from build123d import *

# Parameters (mm, degrees)
BOSS_EXTRUDE1_DEPTH = 18.5
BOSS_EXTRUDE2_DEPTH = 3
BOSS_EXTRUDE3_START = 7
BOSS_EXTRUDE3_DEPTH = 3.5
SKETCH4_W           = 6.5
SKETCH4_H           = 2.25
BOSS_EXTRUDE4_DEPTH = 20
FILLET1_R           = 2.25
BOSS_EXTRUDE5_DEPTH = 7
BOSS_EXTRUDE6_DEPTH = 3
SKETCH7_R           = 2.5
CUT_EXTRUDE1_DEPTH  = 75.541934507
SKETCH8_R           = 2.2
CUT_EXTRUDE2_DEPTH  = 74.11976477
CUT_EXTRUDE3_REACH  = 75.12
SKETCH9_R           = 2.2
BOSS_EXTRUDE7_REACH = 77.196
SKETCH10_R          = 3.5
SKETCH10_R_2        = 2.5
BOSS_EXTRUDE8_REACH = 74.419
SKETCH11_R          = 3.5
SKETCH11_R_2        = 2.5
CUT_EXTRUDE4_REACH  = 66.742
SKETCH12_W          = 7
SKETCH12_H          = 5
CHAMFER1_SIZE       = 1.5


with BuildPart() as part:
    # Sketch1 → Boss-Extrude1 (new body)
    with BuildSketch(Plane(origin=(0, 0, 0), x_dir=(1, 0, 0), z_dir=(0, 1, 0))):
        Polygon((40.5, 0), (0, 0), (0, -58), (3, -58), (3, -3), (40.5, -3), align=None)
    extrude(amount=BOSS_EXTRUDE1_DEPTH)

    # Sketch2 → Boss-Extrude2 (add)
    with BuildSketch(Plane.XZ):
        with BuildLine():
            Line((40.5, 3), (23.5, 19.5))
            Line((23.5, 19.5), (23.5, 37))
            ThreePointArc((23.5, 37), (20.571067812, 44.071067812), (13.5, 47))
            Line((13.5, 47), (3, 47))
            Line((3, 47), (3, 3))
            Line((3, 3), (40.5, 3))
        make_face()
    extrude(amount=-BOSS_EXTRUDE2_DEPTH)

    # Sketch3 → Boss-Extrude3 (add)
    with BuildSketch(Plane(origin=(0, 3, 0), x_dir=(1, 0, 0), z_dir=(0, 1, 0)).offset(BOSS_EXTRUDE3_START)):
        with BuildLine():
            Line((3, -47), (13.5, -47))
            ThreePointArc((13.5, -47), (23.5, -37), (13.5, -27))
            Line((13.5, -27), (3, -27))
            Line((3, -27), (3, -47))
        make_face()
    extrude(amount=BOSS_EXTRUDE3_DEPTH)

    # Sketch4 → Boss-Extrude4 (add)
    with BuildSketch(Plane.XY.offset(47)):
        with Locations((6.25, 14.625)):
            Rectangle(SKETCH4_W, SKETCH4_H)
    extrude(amount=-BOSS_EXTRUDE4_DEPTH)

    # Fillet1
    fillet1_edges = [part.edges().sort_by_distance(p)[0] for p in [
        (9.5, 15.75, 37),
    ]]
    fillet(fillet1_edges, radius=FILLET1_R - 0.0001)  # a hair under: the kernel refuses the full size

    # Sketch5 → Boss-Extrude5 (add)
    with BuildSketch(Plane.XZ):
        Polygon((0, 31.5), (0, 11.5), (9, 11.5), (9, 13.5), (3, 13.5), (3, 31.5), align=None)
    extrude(amount=BOSS_EXTRUDE5_DEPTH)

    # Sketch6 → Boss-Extrude6 (add)
    with BuildSketch(Plane.XZ.offset(7)):
        with BuildLine():
            Line((0, 11.5), (0, 31.5))
            Line((0, 31.5), (13.5, 31.5))
            ThreePointArc((13.5, 31.5), (23.5, 21.5), (13.5, 11.5))
            Line((13.5, 11.5), (0, 11.5))
        make_face()
    extrude(amount=BOSS_EXTRUDE6_DEPTH)

    # Sketch7 → Cut-Extrude1 (cut, through all)
    with BuildSketch(Plane(origin=(0, 13.5, 0), x_dir=(1, 0, 0), z_dir=(0, 1, 0))):
        with Locations(Location((15.5, -21.5, 0), (0, 0, 270))):
            Circle(SKETCH7_R)
        with Locations(Location((15.5, -37, 0), (0, 0, 270))):
            Circle(SKETCH7_R)
    extrude(amount=-CUT_EXTRUDE1_DEPTH, mode=Mode.SUBTRACT)

    # Sketch8 → Cut-Extrude2 (cut, through all)
    with BuildSketch(Plane.ZY):
        with Locations((11, 8.5)):
            Circle(SKETCH8_R)
        with Locations((51.5, 8.5)):
            Circle(SKETCH8_R)
    extrude(amount=-CUT_EXTRUDE2_DEPTH, mode=Mode.SUBTRACT)

    # Sketch9 → Cut-Extrude3 (cut, up to next)
    with BuildSketch(Plane(origin=(0, 0, 0), x_dir=(-1, 0, 0), z_dir=(0, 0, -1)), mode=Mode.PRIVATE) as cut_extrude3_sk1:
        with Locations((-34.5, 8.5)):
            Circle(SKETCH9_R)
    cut_extrude3_tool1 = extrude(cut_extrude3_sk1.sketch, amount=-CUT_EXTRUDE3_REACH, mode=Mode.PRIVATE) & part.part
    # Sketch9 → Cut-Extrude3 (cut, up to next)
    with BuildSketch(Plane(origin=(0, 0, 0), x_dir=(-1, 0, 0), z_dir=(0, 0, -1)), mode=Mode.PRIVATE) as cut_extrude3_sk2:
        with Locations((-11, 8.5)):
            Circle(SKETCH9_R)
    cut_extrude3_tool2 = extrude(cut_extrude3_sk2.sketch, amount=-CUT_EXTRUDE3_REACH, mode=Mode.PRIVATE) & part.part
    add(cut_extrude3_tool1.solids().sort_by_distance((34.5, 8.5, 0))[0], mode=Mode.SUBTRACT)
    add(cut_extrude3_tool2.solids().sort_by_distance((11, 8.5, 0))[0], mode=Mode.SUBTRACT)

    # Sketch10 → Boss-Extrude7 (add, up to next)
    with BuildSketch(Plane(origin=(0, -7, 0), x_dir=(1, 0, 0), z_dir=(0, 1, 0)), mode=Mode.PRIVATE) as boss_extrude7_sk1:
        with Locations(Location((15.5, -21.5, 0), (0, 0, 270))):
            Circle(SKETCH10_R)
        with Locations(Location((15.5, -21.5, 0), (0, 0, 270))):
            Circle(SKETCH10_R_2, mode=Mode.SUBTRACT)
    boss_extrude7_tool1 = extrude(boss_extrude7_sk1.sketch, amount=BOSS_EXTRUDE7_REACH, mode=Mode.PRIVATE) - part.part
    add(boss_extrude7_tool1.solids().sort_by_distance((15.5, -7, 18.098995))[0])

    # Sketch11 → Boss-Extrude8 (add, up to next)
    with BuildSketch(Plane(origin=(0, 3, 0), x_dir=(1, 0, 0), z_dir=(0, 1, 0)), mode=Mode.PRIVATE) as boss_extrude8_sk1:
        with Locations(Location((15.5, -37, 0), (0, 0, 90))):
            Circle(SKETCH11_R)
        with Locations(Location((15.5, -37, 0), (0, 0, 270))):
            Circle(SKETCH11_R_2, mode=Mode.SUBTRACT)
    boss_extrude8_tool1 = extrude(boss_extrude8_sk1.sketch, amount=BOSS_EXTRUDE8_REACH, mode=Mode.PRIVATE) - part.part
    add(boss_extrude8_tool1.solids().sort_by_distance((15.5, 3, 40.401005))[0])

    # Cut-Extrude4: up to this face of the body (flat: up to its plane)
    cut_extrude4_end = Plane(part.part.faces().sort_by_distance((21.694792225, 10.874217494, 3))[0])
    # Sketch12 → Cut-Extrude4 (cut, up to the picked face)
    with BuildSketch(Plane.XY.offset(47), mode=Mode.PRIVATE) as cut_extrude4_sk1:
        with Locations((15.5, -3.5)):
            Rectangle(SKETCH12_W, SKETCH12_H)
    cut_extrude4_tool1 = split(extrude(cut_extrude4_sk1.sketch, amount=-CUT_EXTRUDE4_REACH, mode=Mode.PRIVATE), bisect_by=cut_extrude4_end, keep=Keep.BOTH, mode=Mode.PRIVATE)
    # Sketch12 → Cut-Extrude4 (cut, up to the picked face)
    with BuildSketch(Plane.XY.offset(47), mode=Mode.PRIVATE) as cut_extrude4_sk2:
        with Locations((15.5, 6.5)):
            Rectangle(SKETCH12_W, SKETCH12_H)
    cut_extrude4_tool2 = split(extrude(cut_extrude4_sk2.sketch, amount=-CUT_EXTRUDE4_REACH, mode=Mode.PRIVATE), bisect_by=cut_extrude4_end, keep=Keep.BOTH, mode=Mode.PRIVATE)
    add(cut_extrude4_tool1.solids().sort_by(Axis((15.5, -3.5, 47), (0, 0, -1)))[0], mode=Mode.SUBTRACT)
    add(cut_extrude4_tool2.solids().sort_by(Axis((15.5, 6.5, 47), (0, 0, -1)))[0], mode=Mode.SUBTRACT)

    # Chamfer1
    chamfer1_edges = [part.edges().sort_by_distance(p)[0] for p in [
        (9, -3.5, 13.5),
    ]]
    chamfer(chamfer1_edges, length=CHAMFER1_SIZE)


solid = part.part
Work out the finished part from the listing and answer in its coordinate system (mm). A direction names the side the tool comes from. Coordinates: 2 decimals unless noted, no trailing zeros. Loops run counter-clockwise (first coordinate to the right, second up) from the corner with the lowest first, then second, coordinate; pieces in that order, holes last. Notation, with made-up numbers: M 30.5,43 L 64.5,43 A18 ccw 64.5,57 Z; hole C 52.25,-37.75 d5. An arc over 180 degrees is marked long. Answer in a Markdown table with one row per item. Add a question column.
1. The mould has two halves that part along Y. Classify faces 1 (the cylindrical face through (15.346, 3.493, 40.497)), 2 (the cylindrical face through (8.86, 15.07, 36.86)), 3 (the flat face through (21, 11, 3)): pulls with the +Y half, pulls with the -Y half, needs draft (parallel to the pull), parting line crosses it, or undercut.
2. Flat-ended cylindrical pins translate along their axes: P1, Ø1.5, axis at x = 9, y = 1.5, coming from the +Z side; P2, Ø3, axis at x = 21.5, z = 12.5, coming from the +Y side; P3, Ø0.6, axis at y = -3.5, z = 12, coming from the +X side. Find the tip coordinate at first contact, or state that the pin passes through.
3. Find section B-B, the plane x = 11. Write down the section's boundary in (y, z), then the cut area to 3 significant figures.
4. Find section D-D, the plane y = 11.75. Write down the section's boundary in (x, z).
5. Consider L1, parallel to Y at x = 19, z = 45; L2, parallel to Y at x = 34.5, z = 1.25; L3, parallel to X at y = 10.65, z = 37. Determine where each line is inside the solid, lowest interval first.
6. A tool of negligible diameter and unlimited length cuts with its end or side. For faces 4 (the flat face through (8, 1, 47)), 5 (the flat face through (5, 15.75, 37)), 6 (the cylindrical face through (18.45, -0.51, 23.38)), 7 (the cylindrical face through (23.5, -8.5, 21.7)), 8 (the flat face through (13, 9, 38)), from which of +Z, -Z, +X, -X, +Y, -Y can it reach the whole face along a straight path? Write none if from no direction.
7. Find section A-A, the plane z = 51.5. Write down the section's boundary in (x, y).
8. Find section C-C, the plane z = 21.5. Write down the section's boundary in (x, y), then the cut area to 4 significant figures.
Reported:
| question | item | result |
|---|---|---|
| 1 | face 1 | undercut |
| 1 | face 2 | pulls with the +Y half |
| 1 | face 3 | needs draft |
| 2 | P1 | stops at z = 47 |
| 2 | P2 | stops at y = 3 |
| 2 | P3 | stops at x = 9 |
| 3 | outline | M -10,11.5 L -7,11.5 L -7,31.5 L -10,31.5 Z; M 0,0 L 6.3,0 L 6.3,3 L 3,3 L 3,47 L 0,47 Z; M 10,27 L 13.5,27 L 13.5,47 L 10,47 Z; M 10.7,0 L 18.5,0 L 18.5,3 L 10.7,3 Z |
| 3 | area | 304 mm^2 |
| 4 | outline | M 0,0 L 40.5,0 L 40.5,3 L 3,3 L 3,27 L 13.5,27 A10 ccw 13.5,47 L 3,47 L 3,58 L 0,58 Z; hole C 15.5,37 d5 |
| 5 | L1 | y = 0 to 3, 10 to 13.5 |
| 5 | L2 | y = 0 to 6.3, 10.7 to 18.5 |
| 5 | L3 | x = 0 to 13, 18 to 23.5 |
| 6 | face 4 | +Z, +X, +Y, -Y |
| 6 | face 5 | +Z, +X, +Y |
| 6 | face 6 | none |
| 6 | face 7 | +X, -Y |
| 6 | face 8 | +Z, +X |
| 7 | outline | M 0,0 L 3,0 L 3,6.3 L 0,6.3 Z; M 0,10.7 L 3,10.7 L 3,18.5 L 0,18.5 Z |
| 8 | outline | M 0,-10 L 13,-10 L 13,-6 L 12,-6 L 12,-7 L 3,-7 L 3,0 L 12,0 L 12,-1 L 13,-1 L 13,3 L 3,3 L 3,18.5 L 0,18.5 Z; M 18,-10 L 23.5,-10 L 23.5,-7 L 19,-7 L 19,-6 L 18,-6 Z; M 18,-1 L 19,-1 L 19,0 L 23.5,0 L 23.5,3 L 18,3 Z |
| 8 | area | 182.5 mm^2 |
